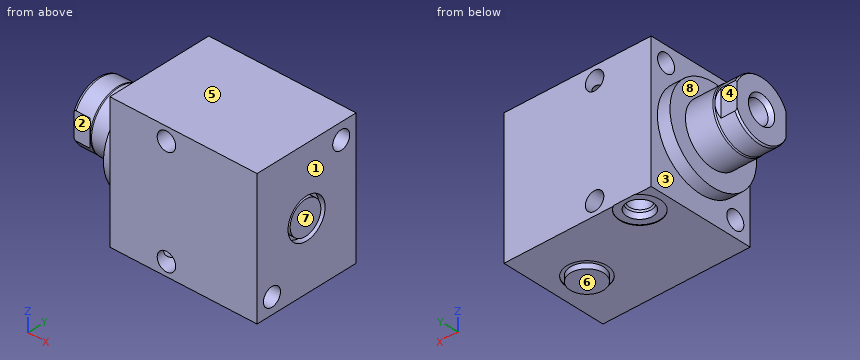
```python
from build123d import *

# Parameters (mm, degrees)
SKETCH1_W          = 63.5
SKETCH1_H          = 50.8
EXTRUDE1_DEPTH     = 69.723
SKETCH5_R          = 22.225
EXTRUDE2_DEPTH     = 5.969
SKETCH6_W          = 14.2875
SKETCH6_H          = 22.86
CUT_EXTRUDE4_DEPTH = 30.48
SKETCH13_R         = 7.874
EXTRUDE3_DEPTH     = 2.54
HOLE1_D            = 8.7376
HOLE1_DEPTH        = 69.723
HOLE2_D            = 8.7376
HOLE2_DEPTH        = 50.8
SKETCH18_R         = 7.874
EXTRUDE4_DEPTH     = 2.54


with BuildPart() as part:
    # Sketch1 → Extrude1 (new body)
    with BuildSketch(Plane(origin=(0, 0, 0), x_dir=(0, 0, -1), z_dir=(1, 0, 0))):
        Rectangle(SKETCH1_W, SKETCH1_H)
    extrude(amount=EXTRUDE1_DEPTH)

    # S2D0002 → Cut-Revolve1 (revolve, cut)
    with BuildSketch(Plane(origin=(0, 17.4498, 0), x_dir=(-1, 0, 0), z_dir=(0, 1, 0)), mode=Mode.PRIVATE) as cut_revolve1_sk:
        Polygon((-18.8849, -31.496), (-22.225, -31.496), (-22.225, -31.75), (-12.7, -31.75), (-12.7, -17.526), (-17.6784, -17.526), (-17.6784, -28.279393135), (-18.342306865, -28.9433), align=None)
    revolve(cut_revolve1_sk.sketch.rotate(Axis((12.7, 17.4498, -19.13842003), (0, 0, 1)), 180), axis=Axis((12.7, 17.4498, -19.13842003), (0, 0, 1)), mode=Mode.SUBTRACT)  # turned: the seam where the file's is

    # Sketch3 → Cut-Revolve2 (revolve, cut)
    with BuildSketch(Plane(origin=(41.148, 0, -25.146), x_dir=(1, 0, 0), z_dir=(0, 1, 0))):
        Polygon((18.8849, 6.35), (22.225, 6.35), (22.225, 6.604), (12.7, 6.604), (12.7, -7.62), (17.6784, -7.62), (17.6784, 3.133393135), (18.342306865, 3.7973), align=None)
    revolve(axis=Axis((53.848, 0, -3.189624441), (0, 0, -1)), mode=Mode.SUBTRACT)

    # Sketch4 → Cut-Revolve3 (revolve, cut)
    with BuildSketch(Plane(origin=(53.975, 0, 0), x_dir=(0, -1, 0), z_dir=(0, 0, 1)), mode=Mode.PRIVATE) as cut_revolve3_sk:
        Polygon((6.1849, 12.7), (9.525, 12.7), (9.525, 15.748), (0, 15.748), (0, 1.3462), (4.9784, 1.3462), (4.9784, 9.483393135), (5.642306865, 10.1473), align=None)
    revolve(cut_revolve3_sk.sketch.rotate(Axis((38.879609832, 0, 0), (1, 0, 0)), 270), axis=Axis((38.879609832, 0, 0), (1, 0, 0)), mode=Mode.SUBTRACT)  # turned: the seam where the file's is

    # Sketch5 → Extrude2 (add)
    with BuildSketch(Plane.ZY):
        Circle(SKETCH5_R)
    extrude(amount=EXTRUDE2_DEPTH)

    # Sketch6 → Revolve1 (revolve)
    with BuildSketch(Plane(origin=(0, 0, 0), x_dir=(0, 0, 1), z_dir=(0, -1, 0)), mode=Mode.PRIVATE) as revolve1_sk:
        with Locations((-7.14375, 17.399)):
            Rectangle(SKETCH6_W, SKETCH6_H)
    revolve(revolve1_sk.sketch.rotate(Axis((5.754582971, 0, 0), (-1, 0, 0)), 180), axis=Axis((5.754582971, 0, 0), (-1, 0, 0)))  # turned: the seam where the file's is

    # S2D0001 → Cut-Revolve4 (revolve, cut)
    with BuildSketch(Plane(origin=(-18.511260017, 3.2639, 0), x_dir=(0, 1, 0), z_dir=(0, 0, 1)), mode=Mode.PRIVATE) as cut_revolve4_sk:
        Polygon((2.286, 8.250017728), (2.286, -6.522460017), (-3.2639, -6.522460017), (-3.2639, 10.317739983), (3.4798, 10.317739983), align=None)
    revolve(cut_revolve4_sk.sketch.rotate(Axis((0, 0, 0), (-1, 0, 0)), 270), axis=Axis((0, 0, 0), (-1, 0, 0)), mode=Mode.SUBTRACT)  # turned: the seam where the file's is

    # Sketch8 → Cut-Revolve5 (revolve, cut)
    with BuildSketch(Plane(origin=(0, 0, 0), x_dir=(0, 0, -1), z_dir=(0, 1, 0)), mode=Mode.PRIVATE) as cut_revolve5_sk:
        with BuildLine():
            Line((-14.2875, 18.923), (-14.097, 19.685))
            Line((-14.097, 19.685), (-14.097, 27.813))
            ThreePointArc((-14.097, 27.813), (-13.996678675, 28.356796865), (-13.708922533, 28.829))
            Line((-13.708922533, 28.829), (-14.2875, 28.829))
            Line((-14.2875, 28.829), (-14.2875, 18.923))
        make_face()
    revolve(cut_revolve5_sk.sketch.rotate(Axis((-12.65936, 0, 0), (-1, 0, 0)), 180), axis=Axis((-12.65936, 0, 0), (-1, 0, 0)), mode=Mode.SUBTRACT)  # turned: the seam where the file's is

    # Sketch12 → Cut-Extrude4 (cut, symmetric)
    with BuildSketch(Plane(origin=(0, 0, 0), x_dir=(0, -1, 0), z_dir=(0, 0, -1))):
        Polygon((12.573, 28.829), (12.573, 21.2598), (14.097, 19.7358), (14.097, 28.829), align=None)
        Polygon((-12.573, 28.829), (-12.573, 21.2598), (-14.097, 19.7358), (-14.097, 28.829), align=None)
    extrude(amount=CUT_EXTRUDE4_DEPTH, both=True, mode=Mode.SUBTRACT)

    # Sketch13 → Extrude3 (add)
    with BuildSketch(Plane(origin=(0, 0, -31.496), x_dir=(-1, 0, 0), z_dir=(0, 0, -1))):
        with Locations(Location((-53.848, 0, 0), (0, 0, 180))):  # turned: the seam where the file's is
            Circle(SKETCH13_R)
    extrude(amount=EXTRUDE3_DEPTH)

    # Hole1
    with Locations(Plane.ZY):
        with Locations((-24.13, -17.78), (24.13, 17.78)):
            Hole(HOLE1_D / 2, depth=HOLE1_DEPTH)

    # Hole2
    with Locations(Plane(origin=(0, 25.4, 0), x_dir=(-1, 0, 0), z_dir=(0, 1, 0))):
        with Locations((-26.797, -25.4), (-26.797, 25.4)):
            Hole(HOLE2_D / 2, depth=HOLE2_DEPTH)

    # Sketch18 → Extrude4 (add)
    with BuildSketch(Plane(origin=(66.675, 0, 0), x_dir=(0, 0, -1), z_dir=(1, 0, 0))):
        with Locations(Location((0, 0, 0), (0, 0, 180))):  # turned: the seam where the file's is
            Circle(SKETCH18_R)
    extrude(amount=EXTRUDE4_DEPTH)


solid = part.part
```
Input: part model. Units: mm. Frame: model coordinates. Face numbers are marked on the shaded views. A direction names the side the tool comes from. Coordinates: 2 decimals unless noted, no trailing zeros. Order: outer loops, then holes, each group sorted by start corner. A loop starts at its lowest first (then second) coordinate and runs counter-clockwise, first axis right, second up. Notation, with made-up numbers: (8, 54.5) - (22, 54.5) arc R26 ccw to (22, 90.5) - close; hole circle Ø1 at (-9, 12). An arc over 180 degrees is marked (long way). Put each result on its own line as item: value.
1. Cut plane C-C on x = 12.7. Return the cut outline in (y, z).
Report:
outline: (-25.4, -31.75) - (7.92, -31.75) - (7.92, -31.5) - (11.26, -31.5) - (11.81, -28.94) - (12.47, -28.28) - (12.47, -17.53) - (22.43, -17.53) - (22.43, -28.28) - (23.09, -28.94) - (23.63, -31.5) - (25.4, -31.5) - (25.4, 31.75) - (-25.4, 31.75) - close; hole circle Ø8.74 at (-17.78, -24.13); hole circle Ø8.74 at (17.78, 24.13)
2. Cut plane B-B on z = -24.13. Return the cut outline in (x, y), then the cut area to 3 significant figures.
Report:
outline: (0, -25.4) - (22.62, -25.4) - (22.62, -22.15) - (0, -22.15) - close; (0, -13.41) - (22.62, -13.41) - (22.62, 25.4) - (0, 25.4) - close; (30.98, -25.4) - (69.72, -25.4) - (69.72, -22.15) - (30.98, -22.15) - close; (30.98, -13.41) - (69.72, -13.41) - (69.72, 25.4) - (30.98, 25.4) - close; hole circle Ø9.96 at (12.7, 17.45); hole circle Ø9.96 at (53.85, 0)
area: 2,430 mm2
3. Draft query along Z for the marked faces 5, 6, 7 and 8. Return one class per face: pulls with the +Z half, pulls with the -Z half, needs draft (parallel to the pull), parting line crosses it, or undercut.
Report:
face 5: pulls with the +Z half
face 6: pulls with the -Z half
face 7: undercut
face 8: needs draft
4. Line query: line 1 along X through (y, z) = (-13.5, -25.5); line 2 along Y through (x, z) = (-22, 0); line 3 along Z through (x, y) = (10.5, 6). Output: solid intervals per line, ascending.
Report:
line 1: x = 0 to 22.43, 31.16 to 69.72
line 2: y = -12.57 to -5.55, 5.55 to 12.57
line 3: z = -31.75 to 31.75
5. Cut plane D-D on z = 24.13. Return the cut outline in (x, y), then the cut area to 3 significant figures.
Report:
outline: (0, -25.4) - (22.62, -25.4) - (22.62, 13.41) - (0, 13.41) - close; (0, 22.15) - (22.62, 22.15) - (22.62, 25.4) - (0, 25.4) - close; (30.98, -25.4) - (69.72, -25.4) - (69.72, 13.41) - (30.98, 13.41) - close; (30.98, 22.15) - (69.72, 22.15) - (69.72, 25.4) - (30.98, 25.4) - close
area: 2,580 mm2
6. Contact query for flat-ended pins moving along their axis: pin 1 Ø1.5 at (y, z) = (0, -8) entering from +X (3 decimals); pin 2 Ø10 at (x, z) = (26.797, -25.4) entering from -Y; pin 3 Ø8.5 at (x, z) = (-23.5, -1) entering from +Y; pin 4 Ø6 at (x, y) = (-9.5, -13.5) entering from +Z. Output: stop coordinate, or through.
Report:
pin 1: stops at x = 69.215
pin 2: stops at y = -25.4
pin 3: stops at y = 14.19
pin 4: stops at z = 9.69
7. Reachability of the marked faces 1, 2, 3 and 4 from +Z, -Z, +X, -X, +Y, -Y: full face, straight path, thin tool, end or side. Return the list, or none.
Report:
face 1: +Z, -Z, +X, +Y, -Y
face 2: +Z, -Z, -X, -Y
face 3: -X
face 4: +Z, -Z, -X, +Y
8. Cut plane A-A on y = -17.78. Return the cut outline in (x, z) (3 decimals), then the cut area to 3 significant figures.
Report:
outline: (-5.969, -13.335) - (0, -13.335) - (0, -19.761) - (69.723, -19.761) - (69.723, 31.75) - (0, 31.75) - (0, 13.335) - (-5.969, 13.335) - close; (0, -31.75) - (69.723, -31.75) - (69.723, -28.499) - (29.877, -28.499) arc R4.369 cw to (23.717, -28.499) - (0, -28.499) - close; hole circle Ø8.738 at (26.797, 25.4)
area: 3,910 mm2
